```python
from build123d import *

# Parameters (mm, degrees)
SKETCH1_W           = 80
SKETCH1_H           = 90
BOSS_EXTRUDE1_DEPTH = 10
SKETCH2_W           = 80
SKETCH2_H           = 70
BOSS_EXTRUDE2_DEPTH = 40
SKETCH3_W           = 59.6
SKETCH3_H           = 14.5
BOSS_EXTRUDE3_DEPTH = 20
CUT_EXTRUDE1_REACH  = 115.578
SKETCH6_W           = 23.6
SKETCH6_H           = 20
CUT_EXTRUDE2_REACH  = 117.434
SKETCH7_W           = 40
SKETCH7_H           = 35
CUT_EXTRUDE3_REACH  = 87
SKETCH8_R           = 2


with BuildPart() as part:
    # Sketch1 → Boss-Extrude1 (new body)
    with BuildSketch(Plane(origin=(0, 0, 0), x_dir=(1, 0, 0), z_dir=(0, 1, 0))):
        Rectangle(SKETCH1_W, SKETCH1_H)
    extrude(amount=BOSS_EXTRUDE1_DEPTH)

    # Sketch2 → Boss-Extrude2 (add)
    with BuildSketch(Plane(origin=(0, 10, 0), x_dir=(1, 0, 0), z_dir=(0, 1, 0))):
        Rectangle(SKETCH2_W, SKETCH2_H)
    extrude(amount=BOSS_EXTRUDE2_DEPTH)

    # Sketch3 → Boss-Extrude3 (add)
    with BuildSketch(Plane(origin=(0, 50, 0), x_dir=(1, 0, 0), z_dir=(0, 1, 0))):
        with Locations((0, -27.75)):
            Rectangle(SKETCH3_W, SKETCH3_H)
        with Locations((0, 27.75)):
            Rectangle(SKETCH3_W, SKETCH3_H)
    extrude(amount=BOSS_EXTRUDE3_DEPTH)

    # Sketch6 → Cut-Extrude1 (cut, up to next)
    with BuildSketch(Plane.XY.offset(35), mode=Mode.PRIVATE) as cut_extrude1_sk1:
        with Locations((0, 60)):
            Rectangle(SKETCH6_W, SKETCH6_H)
    cut_extrude1_tool1 = extrude(cut_extrude1_sk1.sketch, amount=-CUT_EXTRUDE1_REACH, mode=Mode.PRIVATE) & part.part
    add(cut_extrude1_tool1.solids().sort_by_distance((0, 60, 35))[0], mode=Mode.SUBTRACT)

    # Sketch7 → Cut-Extrude2 (cut, up to next)
    with BuildSketch(Plane.ZY.offset(40), mode=Mode.PRIVATE) as cut_extrude2_sk1:
        with Locations((0, 17.5)):
            Rectangle(SKETCH7_W, SKETCH7_H)
    cut_extrude2_tool1 = extrude(cut_extrude2_sk1.sketch, amount=-CUT_EXTRUDE2_REACH, mode=Mode.PRIVATE) & part.part
    add(cut_extrude2_tool1.solids().sort_by_distance((-40, 17.5, 0))[0], mode=Mode.SUBTRACT)

    # Sketch8 → Cut-Extrude3 (cut, up to next)
    with BuildSketch(Plane(origin=(0, 10, 0), x_dir=(1, 0, 0), z_dir=(0, 1, 0)), mode=Mode.PRIVATE) as cut_extrude3_sk1:
        with Locations(Location((-25, -40, 0), (0, 0, 270))):
            Circle(SKETCH8_R)
    cut_extrude3_tool1 = extrude(cut_extrude3_sk1.sketch, amount=-CUT_EXTRUDE3_REACH, mode=Mode.PRIVATE) & part.part
    # Sketch8 → Cut-Extrude3 (cut, up to next)
    with BuildSketch(Plane(origin=(0, 10, 0), x_dir=(1, 0, 0), z_dir=(0, 1, 0)), mode=Mode.PRIVATE) as cut_extrude3_sk2:
        with Locations(Location((25, -40, 0), (0, 0, 270))):
            Circle(SKETCH8_R)
    cut_extrude3_tool2 = extrude(cut_extrude3_sk2.sketch, amount=-CUT_EXTRUDE3_REACH, mode=Mode.PRIVATE) & part.part
    # Sketch8 → Cut-Extrude3 (cut, up to next)
    with BuildSketch(Plane(origin=(0, 10, 0), x_dir=(1, 0, 0), z_dir=(0, 1, 0)), mode=Mode.PRIVATE) as cut_extrude3_sk3:
        with Locations(Location((25, 40, 0), (0, 0, 270))):
            Circle(SKETCH8_R)
    cut_extrude3_tool3 = extrude(cut_extrude3_sk3.sketch, amount=-CUT_EXTRUDE3_REACH, mode=Mode.PRIVATE) & part.part
    # Sketch8 → Cut-Extrude3 (cut, up to next)
    with BuildSketch(Plane(origin=(0, 10, 0), x_dir=(1, 0, 0), z_dir=(0, 1, 0)), mode=Mode.PRIVATE) as cut_extrude3_sk4:
        with Locations(Location((-25, 40, 0), (0, 0, 270))):
            Circle(SKETCH8_R)
    cut_extrude3_tool4 = extrude(cut_extrude3_sk4.sketch, amount=-CUT_EXTRUDE3_REACH, mode=Mode.PRIVATE) & part.part
    add(cut_extrude3_tool1.solids().sort_by_distance((-25, 10, 40))[0], mode=Mode.SUBTRACT)
    add(cut_extrude3_tool2.solids().sort_by_distance((25, 10, 40))[0], mode=Mode.SUBTRACT)
    add(cut_extrude3_tool3.solids().sort_by_distance((25, 10, -40))[0], mode=Mode.SUBTRACT)
    add(cut_extrude3_tool4.solids().sort_by_distance((-25, 10, -40))[0], mode=Mode.SUBTRACT)


solid = part.part
```
Work out the finished part from the listing and answer in its coordinate system (mm). A direction names the side the tool comes from. Give positions to 0.01 mm unless a question says otherwise; leave off trailing zeros. Loops run counter-clockwise (first coordinate to the right, second up) from the corner with the lowest first, then second, coordinate; pieces in that order, holes last. Notation, with made-up numbers: (-39.75, 83.25) -> (-9.75, 83.25) arc R21 ccw to (-9.75, 96.25) -> close; hole circle Ø7 at (47.5, 77). An arc over 180 degrees is marked (long way). Write item = value, one per line. Start each with the question number.
(1) Find the intervals of material crossed by probe 1 along X at (y, z) = (6, -40); probe 2 along Z at (x, y) = (-27.5, 4); probe 3 along Z at (x, y) = (15, 24), in increasing order. Write a range as from..to.
(2) Which of the six approach directions +Z, -Z, +X, -X, +Y, -Y give full straight-line access (tool end or side, diameter ignored) to faces 3 (the flat face through (-11.8, 60, 28)), 4 (the flat face through (-1, 10, -40)), 5 (the flat face through (29.8, 60, -28))?
(3) Find section C-C on x = -19.5. Give the vertices of the cut face in (y, z).
(4) Find section A-A on y = 57.5. Give the vertices of the cut face in (x, z), and give its area (3 significant figures).
(5) Find section B-B on z = -40. Give the vertices of the cut face in (x, y).
(6) Find section D-D on y = 31. Give the vertices of the cut face in (x, z).
(7) The mould has two halves that part along Z. Classify faces 1 (the flat face through (21, 70, 28)), 2 (the cylindrical face through (23.8, 5.1, -41.6)): +Z half, -Z half, draft (parallel to the pull), parting line (faces both ways), or undercut.
(8) Given pin 1 Ø3 at (x, y) = (-23, 31) entering from +Z; pin 2 Ø16 at (y, z) = (59, 30.5) entering from +X; pin 3 Ø7 at (y, z) = (62, -29) entering from -X; pin 4 Ø12 at (y, z) = (10.5, -12) entering from +X, each flat-ended and moving along its own axis, determine where each tip first touches the part or whether it passes through.
From the geometry:
q1.probe_1 = -40..-27, -23..23, 27..40
q1.probe_2 = -45..-20, 20..45
q1.probe_3 = -35..-20, 20..35
q2.face_3 = +Z, +Y
q2.face_4 = -Z, +X, -X, +Y
q2.face_5 = +Z, -Z, +X, +Y
q3.outline = (0, -45) -> (10, -45) -> (10, -35) -> (70, -35) -> (70, -20.5) -> (50, -20.5) -> (50, 20.5) -> (70, 20.5) -> (70, 35) -> (10, 35) -> (10, 45) -> (0, 45) -> (0, 20) -> (35, 20) -> (35, -20) -> (0, -20) -> close
q4.outline = (-29.8, -35) -> (29.8, -35) -> (29.8, -20.5) -> (-29.8, -20.5) -> close; (-29.8, 20.5) -> (-11.8, 20.5) -> (-11.8, 35) -> (-29.8, 35) -> close; (11.8, 20.5) -> (29.8, 20.5) -> (29.8, 35) -> (11.8, 35) -> close
q4.area = 1,390 mm^2
q5.outline = (-40, 0) -> (-27, 0) -> (-27, 10) -> (-40, 10) -> close; (-23, 0) -> (23, 0) -> (23, 10) -> (-23, 10) -> close; (27, 0) -> (40, 0) -> (40, 10) -> (27, 10) -> close
q6.outline = (-40, -35) -> (40, -35) -> (40, -20) -> (-40, -20) -> close; (-40, 20) -> (40, 20) -> (40, 35) -> (-40, 35) -> close
q7.face_1 = draft
q7.face_2 = undercut
q8.pin_1 = 35
q8.pin_2 = 29.8
q8.pin_3 = -29.8
q8.pin_4 = through
